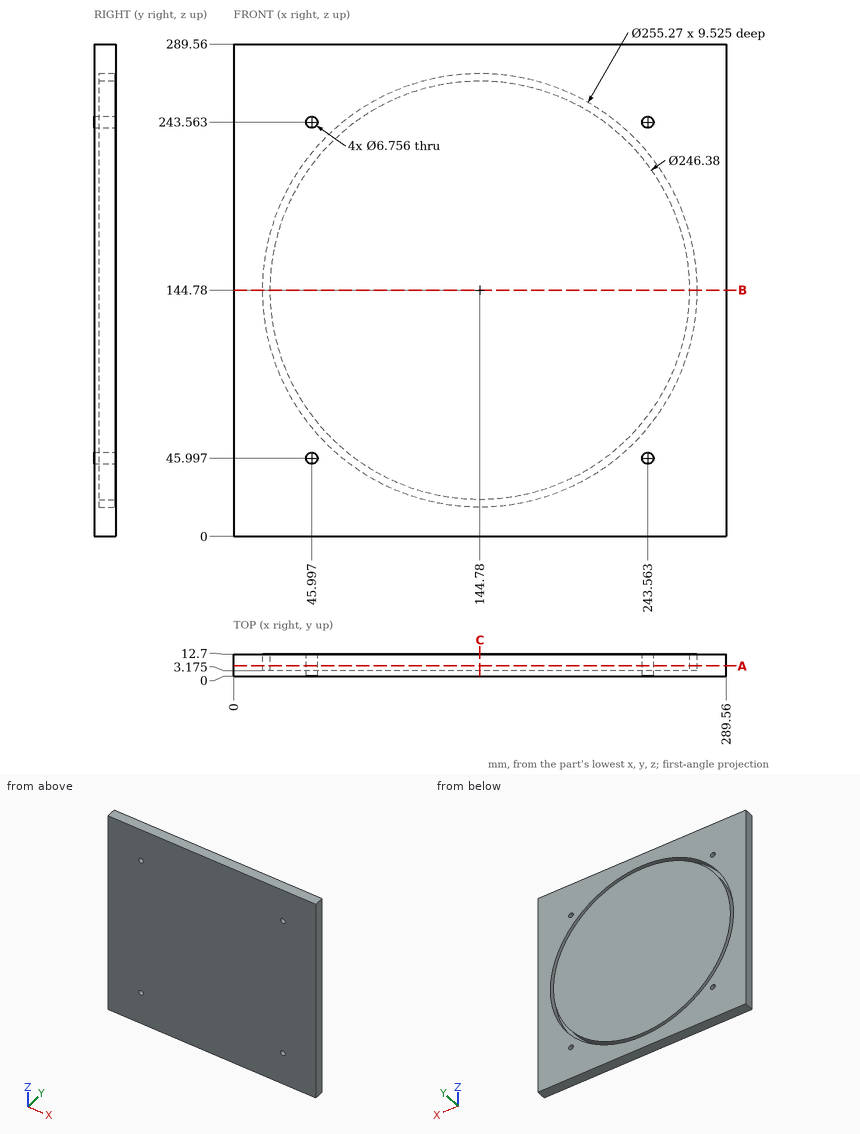
Input: dimensioned drawing with shaded views. Units: mm. Origin: part minimum x, y, z. Round coordinates to 2 decimals unless told otherwise and drop trailing zeros. Order: outer loops, then holes, each group sorted by start corner. A loop starts at its lowest first (then second) coordinate and runs counter-clockwise, first axis right, second up. Notation, with made-up numbers: (51.25, -8.5) - (65.25, -8.5) arc R31 cw to (65.25, 29.5) - close; hole circle Ø1 at (34, 10.25). An arc over 180 degrees is marked (long way). Use CSV: the item, a comma, the result in double quotes. Start each with the question number.
Q1. Section query A-A (y = 6). Return loops of the section in (x, z) (1 decimal).
Q2. Material intervals for line 1 along Z through (x, y) = (144.78, 9) (1 decimal); line 2 along Z through (x, y) = (209, 4.5) (1 decimal); line 3 along X through (y, z) = (7, 108.5), sorted ascending. Write a range as from..to.
Q3. Section query B-B (z = 144.78). Return loops of the section in (x, y) (1 decimal), and give its area (3 significant figures).
Q4. Section query C-C (x = 144.78). Return loops of the section in (y, z) (1 decimal), and give its area (3 significant figures).
Result set:
1,outline,"(0, 0) - (289.6, 0) - (289.6, 289.6) - (0, 289.6) - close; circle Ø246.4 at (144.8, 144.8); hole circle Ø255.3 at (144.8, 144.8); hole circle Ø6.8 at (46, 46); hole circle Ø6.8 at (46, 243.6); hole circle Ø6.8 at (243.6, 46); hole circle Ø6.8 at (243.6, 243.6)"
2,line 1,"z = 0..17.1, 21.6..268, 272.4..289.6"
2,line 2,"z = 0..34.5, 39.7..249.9, 255.1..289.6"
2,line 3,"x = 0..22.41, 27.05..262.51, 267.15..289.56"
3,outline,"(0, 0) - (289.6, 0) - (289.6, 12.7) - (272.4, 12.7) - (272.4, 3.2) - (268, 3.2) - (268, 12.7) - (21.6, 12.7) - (21.6, 3.2) - (17.1, 3.2) - (17.1, 12.7) - (0, 12.7) - close"
3,area,"3,590 mm2"
4,outline,"(0, 0) - (12.7, 0) - (12.7, 17.1) - (3.2, 17.1) - (3.2, 21.6) - (12.7, 21.6) - (12.7, 268) - (3.2, 268) - (3.2, 272.4) - (12.7, 272.4) - (12.7, 289.6) - (0, 289.6) - close"
4,area,"3,590 mm2"
